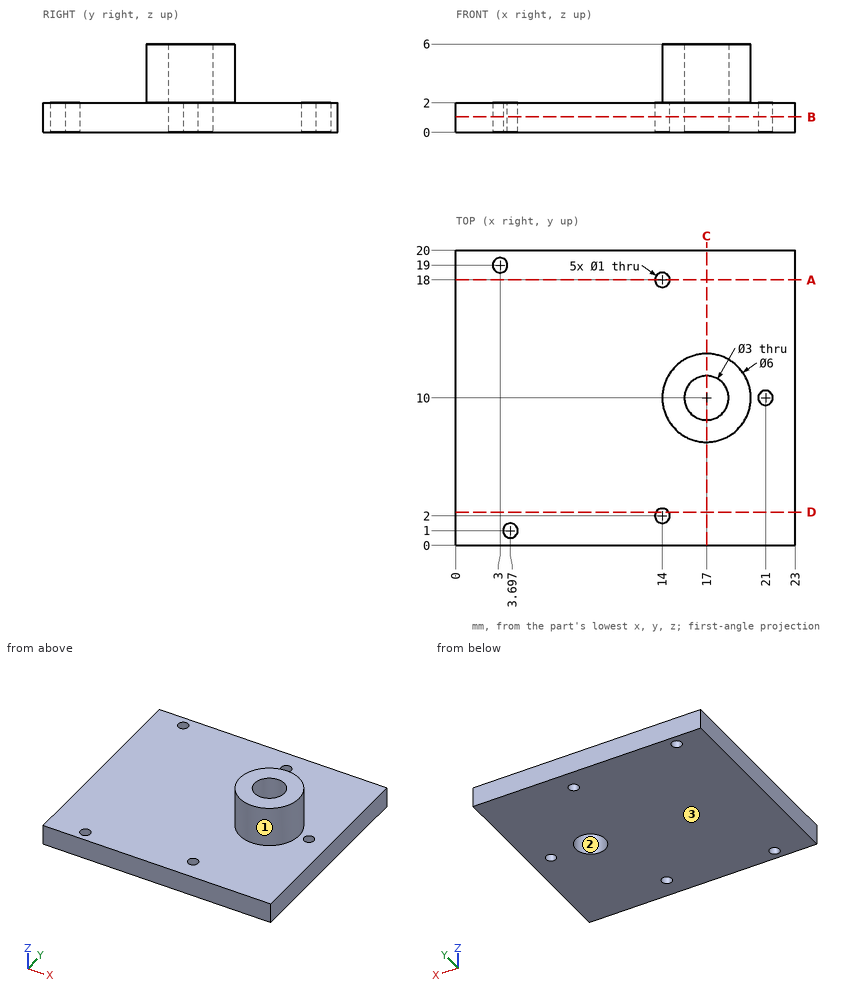
For this review, use the dimensioned drawing (mm, ordinates from the lowest corner) and the shaded views. Give positions to 0.01 mm unless a question says otherwise; leave off trailing zeros. Loops run counter-clockwise (first coordinate to the right, second up) from the corner with the lowest first, then second, coordinate; pieces in that order, holes last.
Item 1: Draft analysis for pull direction X (two halves, no side actions). For the marked faces 1, 2 and 3, state which applies: +X half, -X half, draft (parallel to the pull), parting line (faces both ways), or undercut.
Item 2: Take a section at B-B, the plane z = 1.05. State the section outline as (x, y) points.
Item 3: Take a section at A-A, the plane y = 18. State the section outline as (x, z) points.
Item 4: Take a section at D-D, the plane y = 2.25. State the section outline as (x, z) points, and give its area (3 significant figures).
Item 5: Take a section at C-C, the plane x = 17. State the section outline as (y, z) points.
Item 6: For line 1 along Y through (x, z) = (14, 0.65); line 2 along X through (y, z) = (19, 1.4); line 3 along Y through (x, z) = (3, 0.95), list the stretches that pass through material, from the lowest coordinate up.
Item 7: Insertion check: pin 1 (2.5 mm diameter, centred on x = 17, y = 10, fed in from +Z). The pin has a flat end and moves straight along its axis. Give the tip position at first contact, or say it passes through.
Calculated:
1. face 1: parting line
1. face 2: undercut
1. face 3: draft
2. outline: (0, 0) - (23, 0) - (23, 20) - (0, 20) - close; hole circle Ø1 at (3, 19); hole circle Ø1 at (3.7, 1); hole circle Ø1 at (14, 2); hole circle Ø1 at (14, 18); hole circle Ø3 at (17, 10); hole circle Ø1 at (21, 10)
3. outline: (0, 0) - (13.5, 0) - (13.5, 2) - (0, 2) - close; (14.5, 0) - (23, 0) - (23, 2) - (14.5, 2) - close
4. outline: (0, 0) - (13.57, 0) - (13.57, 2) - (0, 2) - close; (14.43, 0) - (23, 0) - (23, 2) - (14.43, 2) - close
4. area: 44.3 mm2
5. outline: (0, 0) - (8.5, 0) - (8.5, 6) - (7, 6) - (7, 2) - (0, 2) - close; (11.5, 0) - (20, 0) - (20, 2) - (13, 2) - (13, 6) - (11.5, 6) - close
6. line 1: y = 0 to 1.5, 2.5 to 17.5, 18.5 to 20
6. line 2: x = 0 to 2.5, 3.5 to 23
6. line 3: y = 0 to 18.5, 19.5 to 20
7. pin 1: passes through
